Design review of the part built by this model. Coordinates are the model's own, in mm. Face numbers are marked on the shaded views. A direction names the side the tool comes from. Coordinates: 2 decimals unless noted, no trailing zeros. Write each loop counter-clockwise with the first axis right and the second up, starting at its lowest first coordinate (ties: lowest second). Pieces come first, ordered by that corner, then holes.
Q1. Take a section at B-B (z = 0). State how many separate pieces and enclosed holes the cut face has, and give its area (3 significant figures).
Q2. Take a section at C-C (y = -2.75). Give the boundary of the cut face in (x, z) (3 decimals).
Q3. For probe 1 along X at (y, z) = (3.75, -2.5) (3 decimals); probe 2 along Y at (x, z) = (0.15, 0) (3 decimals); probe 3 along X at (y, z) = (-4.75, 2.5), list the stretches that pass through material, from the lowest coordinate up.
Q4. Machinability: for the marked faces 4, 5, 6, 7 and 8, which of the approach directions +Z, -Z, +X, -X, +Y, -Y give a long, thin tool a straight path to every point of the face, cutting with its end or side? Answer none if there is none.
Q5. Insertion check: pin 1 (5 mm diameter, centred on x = 7.5, z = -1.5, fed in from +Y); pin 2 (6 mm diameter, centred on x = 4.5, y = -2, fed in from -Z); pin 3 (1 mm diameter, centred on x = -5.5, z = -3.5, fed in from -Y) (3 decimals). Each pin has a flat end and moves straight along its axis. Give the tip position at first contact, or say it passes through.
Q6. Mouldability with a two-part tool opening along Y and no side actions: class the marked faces 1, 2 and 3 as pulls with the +Y half, pulls with the -Y half, needs draft (parallel to the pull), parting line crosses it, or undercut.
Q7. Take a section at A-A (y = -9). Give the boundary of the cut face in (x, z), and give its area (3 significant figures).
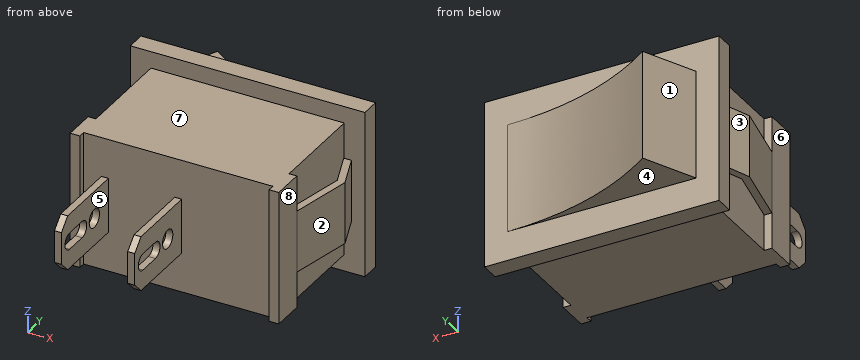
```python
from build123d import *

# Parameters (mm, degrees)
BOSS_EXTRUDE1_DEPTH     = 7.41
CUT_EXTRUDE1_DEPTH      = 15.555353826
CUT_EXTRUDE1_DEPTH_BACK = 15.555353826
SKETCH2_W               = 1.48
SKETCH2_H               = 11.67
BOSS_EXTRUDE2_DEPTH     = 2.75
BOSS_EXTRUDE3_DEPTH     = 4.8125
SKETCH6_R               = 0.820137038
BOSS_EXTRUDE4_DEPTH     = 0.31
LPATTERN1_COUNT         = 2
LPATTERN1_PITCH         = 6.5


with BuildPart() as part:
    # Sketch1 → Boss-Extrude1 (new, symmetric)
    with BuildSketch(Plane.XY):
        Polygon((8.39, -6.985), (9.25, -6.985), (9.25, -4.115), (8.565, -4.115), (8.565, 4.685), (10.4, 4.685), (10.4, 6.385), (-10.4, 6.385), (-10.4, 4.685), (-8.565, 4.685), (-8.565, -4.115), (-9.25, -4.115), (-9.25, -6.985), (-8.39, -6.985), (-8.39, -6.385), (8.39, -6.385), align=None)
    extrude(amount=BOSS_EXTRUDE1_DEPTH, both=True)

    # Sketch2 → Cut-Extrude1 (cut, two sides: drawn at the far end of the back side and taken through both)
    with BuildSketch(Plane(origin=(0, 0, 0), x_dir=(0, 0, -1), z_dir=(1, 0, 0)).offset(-CUT_EXTRUDE1_DEPTH_BACK)):
        with Locations((-6.67, -1.15)):
            Rectangle(SKETCH2_W, SKETCH2_H)
        with Locations((6.67, -1.15)):
            Rectangle(SKETCH2_W, SKETCH2_H)
    extrude(amount=CUT_EXTRUDE1_DEPTH + CUT_EXTRUDE1_DEPTH_BACK, mode=Mode.SUBTRACT)

    # Sketch3 → Boss-Extrude2 (add, symmetric)
    with BuildSketch(Plane.XY):
        Polygon((9.25, -4.115), (10.4, 1.505688207), (9.208432641, 4.685), (8.565, 4.685), (8.565, 4.574090958), (9.715, 1.505688207), (8.565, -4.115), align=None)
        Polygon((-8.565, -4.115), (-9.25, -4.115), (-10.4, 1.505688207), (-9.208432641, 4.685), (-8.565, 4.685), (-8.565, 4.574090958), (-9.715, 1.505688207), align=None)
    extrude(amount=BOSS_EXTRUDE2_DEPTH, both=True)

    # Sketch4 → Boss-Extrude3 (add, symmetric)
    with BuildSketch(Plane.XY):
        with BuildLine():
            Line((-6.210173318, 11.046483266), (-8.365, 6.385))
            Line((-8.365, 6.385), (8.365, 6.385))
            ThreePointArc((8.365, 6.385), (0.713772917, 7.578738259), (-6.210173318, 11.046483266))
        make_face()
    extrude(amount=BOSS_EXTRUDE3_DEPTH, both=True)

    # Sketch6 → Boss-Extrude4 (add, symmetric)
    with BuildSketch(Plane(origin=(0, 0, 0), x_dir=(0, 0, -1), z_dir=(1, 0, 0))):
        Polygon((-2.43, -6.385), (-2.43, -12.885), (-1.43, -13.885), (1.43, -13.885), (2.43, -12.885), (2.43, -6.385), align=None)
        with Locations((0, -8.62789293)):
            Circle(SKETCH6_R, mode=Mode.SUBTRACT)
        with BuildLine():
            Line((0.735277294, -10.583561043), (0.735277294, -12.583561043))
            ThreePointArc((0.735277294, -12.583561043), (0, -13.318838337), (-0.735277294, -12.583561043))
            Line((-0.735277294, -12.583561043), (-0.735277294, -10.583561043))
            ThreePointArc((-0.735277294, -10.583561043), (0, -9.848283749), (0.735277294, -10.583561043))
        make_face(mode=Mode.SUBTRACT)
    boss_extrude4 = extrude(amount=BOSS_EXTRUDE4_DEPTH, both=True)

    # LPattern1: Boss-Extrude4 ×2
    with Locations(*[(-i * LPATTERN1_PITCH, 0, 0) for i in range(1, LPATTERN1_COUNT)]):
        add(boss_extrude4)


solid = part.part
```
Response:
1. separate pieces: 5
1. enclosed holes: 2
1. area: 271 mm2
2. outline: (-9.529, -2.75) - (-8.844, -2.75) - (-8.844, 2.75) - (-9.529, 2.75) - close; (-8.565, -5.93) - (8.565, -5.93) - (8.565, 5.93) - (-8.565, 5.93) - close; (8.844, -2.75) - (9.529, -2.75) - (9.529, 2.75) - (8.844, 2.75) - close
3. probe 1: x = -9.559 to -8.874, -8.565 to 8.565, 8.874 to 9.559
3. probe 2: y = -13.885 to -13.319, -9.848 to -9.448, -7.808 to 7.766
3. probe 3: x = -9.25 to 9.25
4. face 4: -Z, +X, -X, +Y
4. face 5: +Z, -Z, -Y
4. face 6: +Z, -Z, -X, -Y
4. face 7: +Z, +X, -X, -Y
4. face 8: +Z, -Z, +X, -Y
5. pin 1: stops at y = 6.61
5. pin 2: stops at z = -5.93
5. pin 3: stops at y = -6.385
6. face 1: pulls with the +Y half
6. face 2: pulls with the -Y half
6. face 3: undercut
7. outline: (-6.81, -2.43) - (-6.19, -2.43) - (-6.19, -0.73) - (-6.81, -0.73) - close; (-6.81, 0.73) - (-6.19, 0.73) - (-6.19, 2.43) - (-6.81, 2.43) - close; (-0.31, -2.43) - (0.31, -2.43) - (0.31, -0.73) - (-0.31, -0.73) - close; (-0.31, 0.73) - (0.31, 0.73) - (0.31, 2.43) - (-0.31, 2.43) - close
7. area: 4.21 mm2
